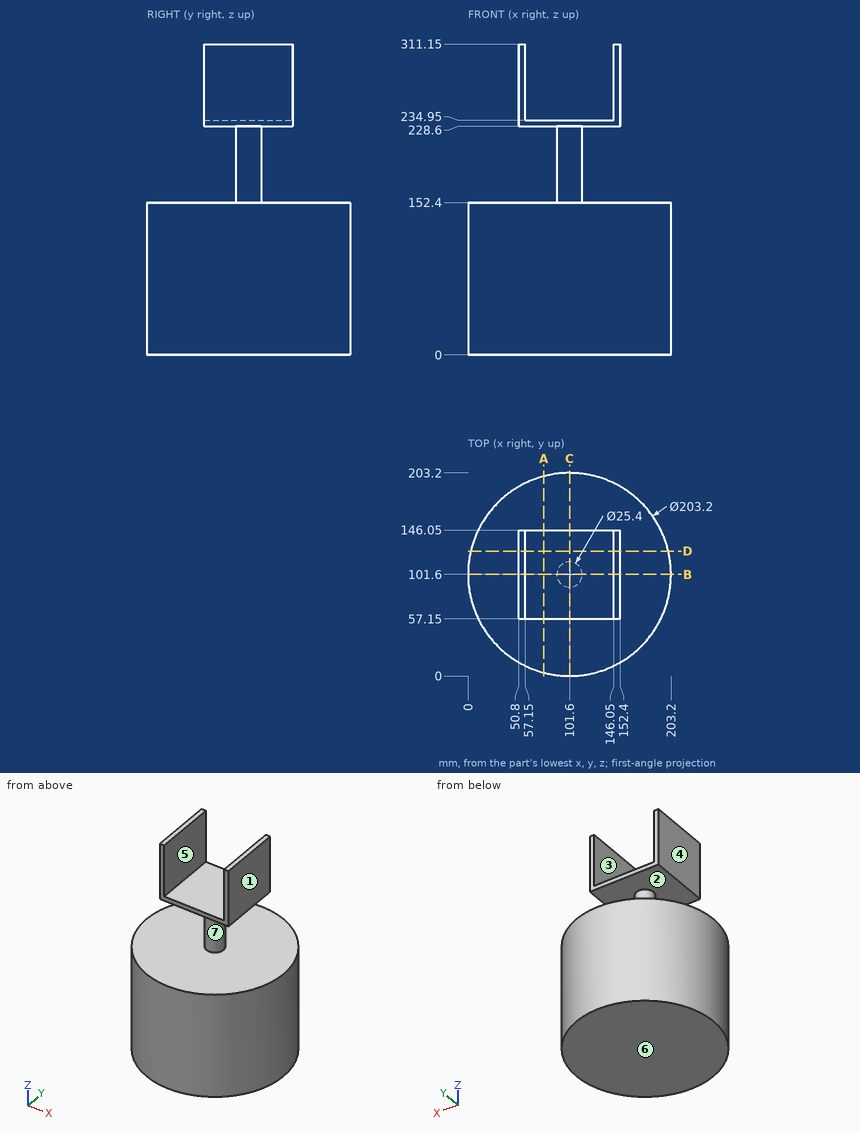
Job drawing, mm, ordinate dimensions from the low corner. One solid piece. A direction names the side the tool comes from. Give positions to 0.01 mm unless a question says otherwise; leave off trailing zeros. Write each loop counter-clockwise with the first axis right and the second up, starting at its lowest first coordinate (ties: lowest second). Pieces come first, ordered by that corner, then holes. Notation, with made-up numbers: M 26.25,88 L 77.25,88 A23 ccw 77.25,113 Z; hole C 43.5,89 d11. An arc over 180 degrees is marked long. Put each result on its own line as item: value. Start each with the question number.
(1) Flat gauge pins, fed straight in: pin 1 Ø6 at (x, z) = (130, 126) entering from -Y; pin 2 Ø4 at (y, z) = (147.5, 111) entering from +X; pin 3 Ø6 at (y, z) = (122.5, 142.5) entering from -X. Where does each tip first touch, or does it go through?
(2) Mould opens along X. For the marked faces 5, 6 and 7 say: +X half, -X half, draft (parallel to the pull), parting line (faces both ways), or undercut.
(3) Which spindle directions (+Z, -Z, +X, -X, +Y, -Y) get a long thin tool onto all of the face, cutting with end or side? Do the marked faces 1, 2, 3 and 4. Say none if no direction does.
(4) Probe L1, parallel to X at y = 135, z = 268.5; L2, parallel to Z at x = 131, y = 70.5; L3, parallel to Z at x = 43.5, y = 95. List the from-to ranges inside material, lowest first.
(5) Band-saw the part on C-C, the plane x = 101.6. Write the cut outline in (y, z), and give its area (3 significant figures).
(6) Band-saw the part on A-A, the plane x = 76. Write the cut outline in (y, z).
(7) Band-saw the part on D-D, the plane y = 125. Write the cut outline in (x, z).
(8) Band-saw the part on B-B, the plane y = 101.6. Write the cut outline in (x, z).
Response values:
1. pin 1: stops at y = 3.23
1. pin 2: stops at x = 193.23
1. pin 3: stops at x = 1.59
2. face 5: undercut
2. face 6: draft
2. face 7: parting line
3. face 1: +Z, +X, +Y, -Y
3. face 2: none
3. face 3: +Z, +Y, -Y
3. face 4: +Z, -X, +Y, -Y
4. L1: x = 50.8 to 57.15, 146.05 to 152.4
4. L2: z = 0 to 152.4, 228.6 to 234.95
4. L3: z = 0 to 152.4
5. outline: M 0,0 L 203.2,0 L 203.2,152.4 L 114.3,152.4 L 114.3,228.6 L 146.05,228.6 L 146.05,234.95 L 57.15,234.95 L 57.15,228.6 L 88.9,228.6 L 88.9,152.4 L 0,152.4 Z
5. area: 33,500 mm2
6. outline: M 3.28,0 L 199.92,0 L 199.92,152.4 L 3.28,152.4 Z; M 57.15,228.6 L 146.05,228.6 L 146.05,234.95 L 57.15,234.95 Z
7. outline: M 2.73,0 L 200.47,0 L 200.47,152.4 L 2.73,152.4 Z; M 50.8,228.6 L 152.4,228.6 L 152.4,311.15 L 146.05,311.15 L 146.05,234.95 L 57.15,234.95 L 57.15,311.15 L 50.8,311.15 Z
8. outline: M 0,0 L 203.2,0 L 203.2,152.4 L 114.3,152.4 L 114.3,228.6 L 152.4,228.6 L 152.4,311.15 L 146.05,311.15 L 146.05,234.95 L 57.15,234.95 L 57.15,311.15 L 50.8,311.15 L 50.8,228.6 L 88.9,228.6 L 88.9,152.4 L 0,152.4 Z
